from build123d import *

# Parameters (mm, degrees)
SKETCH_1_R             = 1.5
EXTRUDE_1_DEPTH        = 1.5
EXTRUDE_2_DEPTH        = 2
SKETCH_4_W             = 0.7
SKETCH_4_H             = 0.7
EXTRUDE_3_DEPTH        = 1
EXTRUDE_4_DEPTH        = 0.7
PATTERN_LINEAR_1_COUNT = 3
PATTERN_LINEAR_1_PITCH = 2.54
CHAMFER_1_SIZE         = 0.2


with BuildPart() as part:
    # 草图1 → 凸台-拉伸1 (new body)
    with BuildSketch(Plane.XY):
        Polygon((-10.05, -29.9), (10.05, -29.9), (10.05, 12.1), (7.05, 15.1), (7.05, 21.9), (10.05, 24.9), (10.05, 29.9), (-10.05, 29.9), (-10.05, 24.9), (-7.05, 21.9), (-7.05, 15.1), (-10.05, 12.1), align=None)
        with Locations((7.55, 27.4)):
            Circle(SKETCH_1_R, mode=Mode.SUBTRACT)
        with Locations(Location((-7.55, 27.4, 0), (0, 0, 180))):
            Circle(SKETCH_1_R, mode=Mode.SUBTRACT)
    extrude(amount=EXTRUDE_1_DEPTH)

    # 草图3 → 凸台-拉伸2 (add)
    with BuildSketch(Plane.XY.offset(1.5)):
        Polygon((-3.456446609, 29), (-3.81, 28.646446609), (-3.81, 26.813553391), (-3.456446609, 26.46), (-1.623553391, 26.46), (-1.27, 26.813553391), (-0.916446609, 26.46), (0.916446609, 26.46), (1.27, 26.813553391), (1.623553391, 26.46), (3.456446609, 26.46), (3.81, 26.813553391), (3.81, 28.646446609), (3.456446609, 29), (1.623553391, 29), (1.27, 28.646446609), (0.916446609, 29), (-0.916446609, 29), (-1.27, 28.646446609), (-1.623553391, 29), align=None)
    extrude(amount=EXTRUDE_2_DEPTH)

    # 草图4 → 凸台-拉伸3 (add)
    with BuildSketch(Plane.XY.offset(3.5)):
        with Locations((-2.54, 27.73)):
            Rectangle(SKETCH_4_W, SKETCH_4_H)
        with Locations((0, 27.73)):
            Rectangle(SKETCH_4_W, SKETCH_4_H)
        with Locations((2.54, 27.73)):
            Rectangle(SKETCH_4_W, SKETCH_4_H)
    extrude(amount=EXTRUDE_3_DEPTH)

    # 草图5 → 凸台-拉伸4 (add)
    with BuildSketch(Plane(origin=(2.89, 0, 0), x_dir=(0, 0, -1), z_dir=(1, 0, 0))):
        with BuildLine():
            Line((-3.5, 27.38), (-4.5, 27.38))
            ThreePointArc((-4.5, 27.38), (-5.045144747, 27.605806348), (-5.270951094, 28.150951094))
            Line((-5.270951094, 28.150951094), (-5.270951094, 35.150951094))
            Line((-5.270951094, 35.150951094), (-4.570951094, 35.150951094))
            Line((-4.570951094, 35.150951094), (-4.570951094, 28.150951094))
            ThreePointArc((-4.570951094, 28.150951094), (-4.55017, 28.100781094), (-4.5, 28.08))
            Line((-4.5, 28.08), (-3.5, 28.08))
            Line((-3.5, 28.08), (-3.5, 27.38))
        make_face()
    extrude_4 = extrude(amount=-EXTRUDE_4_DEPTH)

    # 阵列(线性)1: 凸台-拉伸4 ×3
    with Locations(*[(-i * PATTERN_LINEAR_1_PITCH, 0, 0) for i in range(1, PATTERN_LINEAR_1_COUNT)]):
        add(extrude_4)

    # 倒角1
    chamfer_1_edges = [part.edges().sort_by_distance(p)[0] for p in [
        (2.89, 35.150951094, 4.920951094),
        (2.19, 35.150951094, 4.920951094),
        (2.54, 35.150951094, 5.270951094),
        (2.54, 35.150951094, 4.570951094),
        (0.35, 35.150951094, 4.920951094),
        (-0.35, 35.150951094, 4.920951094),
        (0, 35.150951094, 5.270951094),
        (0, 35.150951094, 4.570951094),
        (-2.89, 35.150951094, 4.920951094),
        (-2.54, 35.150951094, 5.270951094),
        (-2.54, 35.150951094, 4.570951094),
        (-2.19, 35.150951094, 4.920951094),
    ]]
    chamfer(chamfer_1_edges, length=CHAMFER_1_SIZE)


solid = part.part
Design review of the part built by this model. Coordinates are the model's own, in mm. A direction names the side the tool comes from. Coordinates: 2 decimals unless noted, no trailing zeros. Loops run counter-clockwise (first coordinate to the right, second up) from the corner with the lowest first, then second, coordinate; pieces in that order, holes last. Notation, with made-up numbers: (24.25, 17.5) -> (29.25, 17.5) arc R24 ccw to (29.25, 47.5) -> close; hole circle Ø1 at (-38, -3.75). An arc over 180 degrees is marked (long way). Use a Markdown table: item, result. Add a question column.
Item 1: The part is to be moulded in two halves that separate along Z. For faces 1 (the flat face through (3, 29, 2)), 2 (the cylindrical face through (-7.225, 28.864, 0.74)), say which applies: +Z half, -Z half, draft (parallel to the pull), parting line (faces both ways), or undercut.
Item 2: Clearance check with flat-ended pins moving along their axes: P1, Ø1.4, axis at y = 31, z = 4.5, coming from the +X side; P2, Ø1.5, axis at x = 0.5, z = 2, coming from the +Y side; P3, Ø0.6, axis at x = -2.5, z = 4, coming from the -Y side. State where each tip first meets the part, or that it passes through.
Item 3: Wall thickness on L1, parallel to Z at x = -0.75, y = -20; L2, parallel to Y at x = -7.55, z = 0.4; L3, parallel to Y at x = -7.5, z = 0.9: over which ranges is each line inside the solid? List them lowest first. Write a range as from..to.
Item 4: Machinability: for faces 3 (the flat face through (8.53, 23.38, 0.74)), 4 (the flat face through (0, 26.46, 2)), 5 (the flat face through (-7.05, 19, 1)), 6 (the flat face through (-3, 29, 2)), 7 (the flat face through (3.81, 28, 2)), which of the approach directions +Z, -Z, +X, -X, +Y, -Y give a long, thin tool a straight path to every point of the face, cutting with its end or side? Answer none if there is none.
Item 5: We need section A-A, the plane y = 4.5. Write out the cut boundary in (x, z), and give its area (4 significant figures).
Numbers:
| question | item | result |
|---|---|---|
| 1 | face 1 | undercut |
| 1 | face 2 | draft |
| 2 | P1 | stops at x = 2.89 |
| 2 | P2 | stops at y = 29.9 |
| 2 | P3 | stops at y = 27.38 |
| 3 | L1 | z = 0..1.5 |
| 3 | L2 | y = -29.9..14.6, 22.4..25.9, 28.9..29.9 |
| 3 | L3 | y = -29.9..14.65, 22.35..25.9, 28.9..29.9 |
| 4 | face 3 | +Z, -Z, +X |
| 4 | face 4 | +Z, +X, -X, -Y |
| 4 | face 5 | +Z, -Z, -X |
| 4 | face 6 | +X, -X, +Y |
| 4 | face 7 | +Z, +X, +Y, -Y |
| 5 | outline | (-10.05, 0) -> (10.05, 0) -> (10.05, 1.5) -> (-10.05, 1.5) -> close |
| 5 | area | 30.15 mm^2 |
